Read the model definition and answer for the solid it produces. Units are mm, in the model's axes. Coordinates: 2 decimals unless noted, no trailing zeros. Write each loop counter-clockwise with the first axis right and the second up, starting at its lowest first coordinate (ties: lowest second). Pieces come first, ordered by that corner, then holes. Notation, with made-up numbers: (49, -17) -> (67, -17) arc R28 ccw to (67, 11) -> close; hole circle Ø6 at (39, 31.5). An arc over 180 degrees is marked (long way). Return JSON: item names as keys, results as strings.
from build123d import *

# Parameters (mm, degrees)
F0_R     = 2.5
F1_DEPTH = 40
F4_DEPTH = 12.5
F5_DEPTH = 12.5


with BuildPart() as f1:
    # F0 (on Front) → F1 (new body, symmetric)
    with BuildSketch(Plane.XZ):
        Circle(F0_R)
    extrude(amount=F1_DEPTH, both=True)

    # F3 (on Top) → F4 (cut, symmetric)
    with BuildSketch(Plane.XY):
        Polygon((0, -40.4892601073), (-4.2708204128, -31.7243561149), (-4.5337388292, -41.365750134), (5.0189574249, -41.1904491484), (5.2598807418, -31.7243561149), (4.0549240075, -31.1984587461), align=None)
    extrude(amount=F4_DEPTH, both=True, mode=Mode.SUBTRACT)

    # F2 (on Top) → F5 (cut, symmetric)
    with BuildSketch(Plane.XY):
        Polygon((-3.1360695139, 40.8483743668), (-3.1360695139, 33.1261791289), (0, 40.0613993406), (3.1597327907, 33.1261791289), (3.4056627192, 40.8483743668), align=None)
    extrude(amount=F5_DEPTH, both=True, mode=Mode.SUBTRACT)


solid = f1.part
1. Flat-ended cylindrical pins translate along their axes: pin 1 Ø1.5 at (x, y) = (-1.5, 4.5) entering from -Z; pin 2 Ø1.5 at (y, z) = (-11, -1.5) entering from -X. Find the tip coordinate at first contact, or state that the pin passes through.
Taken from the geometry:
{"pin 1": "stops at z = -2.38", "pin 2": "stops at x = -2.38"}
2. The part is cut by section B-B (y = -1). Determine the outline of the cut face in (x, z), then the cut area to 3 significant figures.
Taken from the geometry:
{"outline": "circle Ø5 at (0, 0)", "area": "19.6 mm2"}
3. Consider L1, parallel to X at y = 18.5, z = -0.1; L2, parallel to Z at x = -0.45, y = 17; L3, parallel to Y at x = -2.15, z = -1. Determine where each line is inside the solid, lowest interval first.
Taken from the geometry:
{"L1": "x = -2.5 to 2.5", "L2": "z = -2.46 to 2.46", "L3": "y = -36.08 to 35.31"}
4. The part is cut by section C-C (x = 1.1). Determine the outline of the cut face in (y, z) (3 decimals).
Taken from the geometry:
{"outline": "(-37.969, -2.245) -> (37.647, -2.245) -> (37.647, 2.245) -> (-37.969, 2.245) -> close"}
5. The part is cut by section A-A (z = 0). Determine the outline of the cut face in (x, y), then the cut area to 3 significant figures.
Taken from the geometry:
{"outline": "(-2.5, -35.36) -> (-0.24, -40) -> (0.21, -40) -> (2.5, -34.76) -> (2.5, 34.57) -> (0.03, 40) -> (-0.03, 40) -> (-2.5, 34.53) -> close", "area": "375 mm2"}
